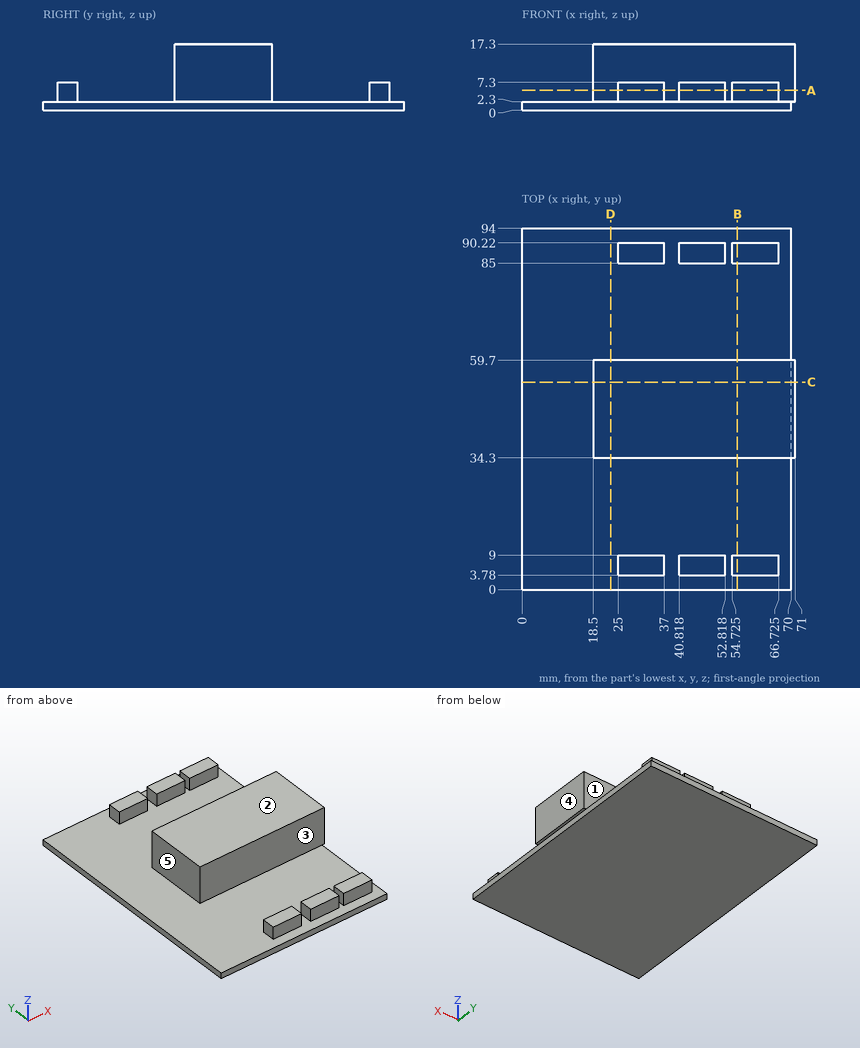
Job drawing, mm, ordinate dimensions from the low corner. One solid piece. A direction names the side the tool comes from. Round coordinates to 2 decimals unless told otherwise and drop trailing zeros. Write each loop counter-clockwise with the first axis right and the second up, starting at its lowest first coordinate (ties: lowest second). Pieces come first, ordered by that corner, then holes.
1) Band-saw the part on A-A, the plane z = 5.25. List the corners of the cut face in (x, y) (1 decimal), and give its area (3 significant figures).
2) Mould opens along Y. For the marked faces 1, 2 and 3 say: +Y half, -Y half, draft (parallel to the pull), parting line (faces both ways), or undercut.
3) Band-saw the part on C-C, the plane y = 54. List the corners of the cut face in (x, z).
4) Pin check, flat tips, straight feed: pin 1 (2.5 mm diameter, centred on x = 47.5, y = 87, fed in from +Z); pin 2 (1.5 mm diameter, centred on x = 49.5, z = 5, fed in from +Y); pin 3 (1 mm diameter, centred on x = 49.5, z = 9.5, fed in from +Y). Stop position of each tip, or through.
5) 3-axis set-ups, long thin cutter, end or side, ignore diameter. For the marked faces 4 and 5: which of +Z, -Z, +X, -X, +Y, -Y reach the whole face in a straight line?
6) Drill centre lines: probe 1 along Z at (x, y) = (46, 20.5); probe 2 along X at (y, z) = (49, 14); probe 3 along Y at (x, z) = (26, 8.5). Where is each one in solid material? Low to high.
7) Band-saw the part on B-B, the plane x = 56. List the corners of the cut face in (y, z).
8) Band-saw the part on D-D, the plane x = 23. List the corners of the cut face in (y, z), and give its area (3 significant figures).
Ans:
1. outline: (18.5, 34.3) - (71, 34.3) - (71, 59.7) - (18.5, 59.7) - close; (25, 3.8) - (37, 3.8) - (37, 9) - (25, 9) - close; (25, 85) - (37, 85) - (37, 90.2) - (25, 90.2) - close; (40.8, 3.8) - (52.8, 3.8) - (52.8, 9) - (40.8, 9) - close; (40.8, 85) - (52.8, 85) - (52.8, 90.2) - (40.8, 90.2) - close; (54.7, 3.8) - (66.7, 3.8) - (66.7, 9) - (54.7, 9) - close; (54.7, 85) - (66.7, 85) - (66.7, 90.2) - (54.7, 90.2) - close
1. area: 1,710 mm2
2. face 1: undercut
2. face 2: draft
2. face 3: undercut
3. outline: (0, 0) - (70, 0) - (70, 2.3) - (71, 2.3) - (71, 17.3) - (18.5, 17.3) - (18.5, 2.3) - (0, 2.3) - close
4. pin 1: stops at z = 7.3
4. pin 2: stops at y = 90.22
4. pin 3: stops at y = 59.7
5. face 4: +Z, -Z, +X, +Y, -Y
5. face 5: +Z, -X, +Y, -Y
6. probe 1: z = 0 to 2.3
6. probe 2: x = 18.5 to 71
6. probe 3: y = 34.3 to 59.7
7. outline: (0, 0) - (94, 0) - (94, 2.3) - (90.22, 2.3) - (90.22, 7.3) - (85, 7.3) - (85, 2.3) - (59.7, 2.3) - (59.7, 17.3) - (34.3, 17.3) - (34.3, 2.3) - (9, 2.3) - (9, 7.3) - (3.78, 7.3) - (3.78, 2.3) - (0, 2.3) - close
8. outline: (0, 0) - (94, 0) - (94, 2.3) - (59.7, 2.3) - (59.7, 17.3) - (34.3, 17.3) - (34.3, 2.3) - (0, 2.3) - close
8. area: 597 mm2
